```python
from build123d import *

# Parameters (mm, degrees)
SKETCH1_R           = 2.6
SKETCH1_R_2         = 2.1
SKETCH1_R_3         = 4.2
SKETCH1_R_4         = 2.5
BOSS_EXTRUDE1_DEPTH = 12
FILLET2_R           = 6
FILLET3_R           = 3
CUT_EXTRUDE1_DEPTH  = 13
SKETCH5_R           = 4
CUT_EXTRUDE2_DEPTH  = 13
SKETCH6_R           = 14.5
CUT_EXTRUDE3_DEPTH  = 6
FILLET4_R           = 12
SKETCH7_R           = 2.6
CUT_EXTRUDE4_DEPTH  = 13
FILLET6_R           = 3
FILLET8_R           = 5
FILLET9_R           = 4
CUT_EXTRUDE6_DEPTH  = 13
FILLET10_R          = 4


with BuildPart() as part:
    # Sketch1 → Boss-Extrude1 (new body)
    with BuildSketch(Plane(origin=(0, 0, 0), x_dir=(1, 0, 0), z_dir=(0, 1, 0))):
        Polygon((162, 19), (137, 30), (83.968719423, 30), (78.968719423, 34), (13.968719423, 52), (17, 87), (9, 87), (-2, 53), (-14, 14), (-14, 2), (-14, -1), (-6, -1), (0, 0), (137, 0), (162, 7), align=None)
        with Locations((-7, 10)):
            Circle(SKETCH1_R, mode=Mode.SUBTRACT)
        with Locations((157, 13)):
            Circle(SKETCH1_R, mode=Mode.SUBTRACT)
        with Locations((5, 26)):
            Circle(SKETCH1_R_2, mode=Mode.SUBTRACT)
        with Locations((9, 41)):
            Circle(SKETCH1_R_3, mode=Mode.SUBTRACT)
        with Locations((143, 13)):
            Circle(SKETCH1_R_4, mode=Mode.SUBTRACT)
    extrude(amount=BOSS_EXTRUDE1_DEPTH)

    # Fillet2
    fillet2_edges = [part.edges().sort_by_distance(p)[0] for p in [
        (137, 6, -30),
        (162, 6, -19),
        (162, 6, -7),
        (137, 6, 0),
    ]]
    fillet(fillet2_edges, radius=FILLET2_R)

    # Fillet3
    fillet3_edges = [part.edges().sort_by_distance(p)[0] for p in [
        (9, 6, -87),
        (17, 6, -87),
    ]]
    fillet(fillet3_edges, radius=FILLET3_R)

    # Sketch4 → Cut-Extrude1 (cut, through all)
    with BuildSketch(Plane(origin=(0, 12, 0), x_dir=(1, 0, 0), z_dir=(0, 1, 0))):
        Polygon((21, 42), (21, 24), (46, 24), (46, 36), align=None)
        Polygon((97, 23.043498828), (83, 23.043498828), (83, 7), (101, 7), align=None)
    extrude(amount=-CUT_EXTRUDE1_DEPTH, mode=Mode.SUBTRACT)

    # Sketch5 → Cut-Extrude2 (cut, through all)
    with BuildSketch(Plane(origin=(0, 12, 0), x_dir=(1, 0, 0), z_dir=(0, 1, 0))):
        with Locations((63, 18)):
            Circle(SKETCH5_R)
    extrude(amount=-CUT_EXTRUDE2_DEPTH, mode=Mode.SUBTRACT)

    # Sketch6 → Cut-Extrude3 (cut)
    with BuildSketch(Plane(origin=(0, 12, 0), x_dir=(1, 0, 0), z_dir=(0, 1, 0))):
        with Locations((63, 18)):
            Circle(SKETCH6_R)
    extrude(amount=-CUT_EXTRUDE3_DEPTH, mode=Mode.SUBTRACT)

    # Fillet4
    fillet4_edges = [part.edges().sort_by_distance(p)[0] for p in [
        (13.968719423, 6, -52),
        (83.968719423, 6, -30),
    ]]
    fillet(fillet4_edges, radius=FILLET4_R)

    # Sketch7 → Cut-Extrude4 (cut, through all)
    with BuildSketch(Plane(origin=(0, 12, 0), x_dir=(1, 0, 0), z_dir=(0, 1, 0))):
        with Locations((47, 6)):
            Circle(SKETCH7_R)
    extrude(amount=-CUT_EXTRUDE4_DEPTH, mode=Mode.SUBTRACT)

    # Fillet6
    fillet6_edges = [part.edges().sort_by_distance(p)[0] for p in [
        (97, 6, -23.043498828),
        (101, 6, -7),
        (83, 6, -7),
        (83, 6, -23.043498828),
    ]]
    fillet(fillet6_edges, radius=FILLET6_R)

    # Fillet8
    fillet8_edges = [part.edges().sort_by_distance(p)[0] for p in [
        (-14, 6, 1),
    ]]
    fillet(fillet8_edges, radius=FILLET8_R)

    # Fillet9
    fillet9_edges = [part.edges().sort_by_distance(p)[0] for p in [
        (21, 6, -42),
        (46, 6, -36),
        (46, 6, -24),
        (21, 6, -24),
    ]]
    fillet(fillet9_edges, radius=FILLET9_R)

    # Sketch10 → Cut-Extrude6 (cut, through all)
    with BuildSketch(Plane(origin=(0, 12, 0), x_dir=(1, 0, 0), z_dir=(0, 1, 0))):
        Polygon((103, 30), (107, 16), (136, 16), (136, 30), align=None)
    extrude(amount=-CUT_EXTRUDE6_DEPTH, mode=Mode.SUBTRACT)

    # Fillet10
    fillet10_edges = [part.edges().sort_by_distance(p)[0] for p in [
        (103, 6, -30),
        (136, 6, -16),
        (107, 6, -16),
    ]]
    fillet(fillet10_edges, radius=FILLET10_R)


solid = part.part
```
Input: part model. Units: mm. Frame: model coordinates. A direction names the side the tool comes from. Coordinates: 2 decimals unless noted, no trailing zeros. Loops run counter-clockwise (first coordinate to the right, second up) from the corner with the lowest first, then second, coordinate; pieces in that order, holes last. Notation, with made-up numbers: M -38,16 L -12,16 A3 cw -12,20 Z; hole C 82,-33 d8. An arc over 180 degrees is marked long. One line per item, written item: value.
(1) Pull-direction query (Z, two-part tool) for faces 5 (the flat face through (-3, 5.9, 0.5)), 6 (the cylindrical face through (83.86, 5.92, -7.9)), 7 (the cylindrical face through (102.363, 5.916, -29.215)); classes: +Z half, -Z half, draft (parallel to the pull), parting line (faces both ways), or undercut.
Filled in:
face 5: +Z half
face 6: undercut
face 7: -Z half
(2) Section C-C (y = 4.25). Give the number of separate pieces and of enclosed holes in the cut face, and give its area (3 significant figures).
Filled in:
separate pieces: 1
enclosed holes: 9
area: 5,500 mm^2
(3) Reachability of faces 1 (the flat face through (94, 6, -30)), 2 (the flat face through (34.55, 6.08, -38.75)), 3 (the flat face through (105, 6, -23)), 4 (the cylindrical face through (48.514, 9.042, -18.638)) from +Z, -Z, +X, -X, +Y, -Y: full face, straight path, thin tool, end or side. Return the list, or none.
Filled in:
face 1: -Z, +X, +Y, -Y
face 2: +Y, -Y
face 3: -Z, +Y, -Y
face 4: +Y
(4) Section D-D (z = -72.5). Output: boundary loops of the cut face in (x, y).
Filled in:
outline: M 4.31,0 L 15.74,0 L 15.74,12 L 4.31,12 Z
(5) Line query: line 1 along X through (y, z) = (6.75, -13); line 2 along X through (y, z) = (8.25, -10); line 3 along X through (y, z) = (6.75, -22). Output: solid intervals per line, ascending. Write a range as from..to.
Filled in:
line 1: -14..49.39, 76.61..83, 99.5..140.5, 145.5..154.4, 159.6..162
line 2: -14..-9.6, -4.4..50.91, 75.09..83, 100.16..161.8
line 3: -11.54..49.06, 76.94..83.73, 96.93..105.29, 136..155.18
(6) Section A-A (x = 143). Output: boundary loops of the cut face in (y, z).
Filled in:
outline: M 0,-27.36 L 12,-27.36 L 12,-15.5 L 0,-15.5 Z; M 0,-10.5 L 12,-10.5 L 12,-1.68 L 0,-1.68 Z
(7) Section B-B (x = 124). Output: boundary loops of the cut face in (y, z).
Filled in:
outline: M 0,-16 L 12,-16 L 12,0 L 0,0 Z
(8) Pin query (flat end, axial travel): pin 1 (5 mm diameter, centred on x = 131.5, y = 5, fed in from -Z); pin 2 (5.5 mm diameter, centred on y = 6, z = -30.5, fed in from -X); pin 3 (6 mm diameter, centred on x = 88, y = 8, fed in from +Z). Return the tip coordinate at first contact, or that it passes through.
Filled in:
pin 1: z = -16.54
pin 2: x = -9.77
pin 3: z = 0
